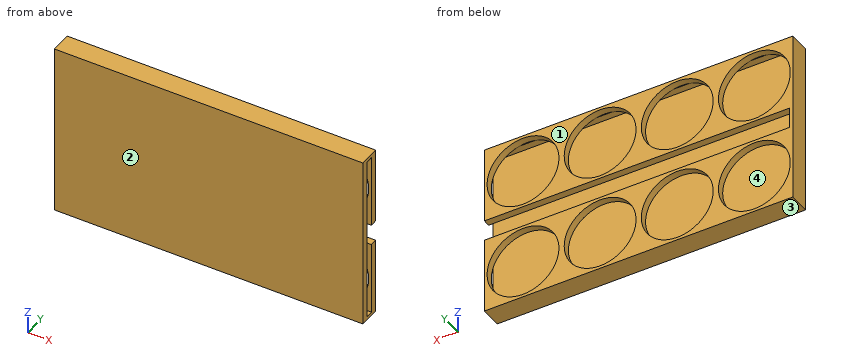
from build123d import *

# Parameters (mm, degrees)
SKETCH1_W           = 88
SKETCH1_H           = 50
BOSS_EXTRUDE1_DEPTH = 6
SKETCH2_W           = 48
SKETCH2_H           = 2
CUT_EXTRUDE1_DEPTH  = 87
SKETCH3_R           = 10.25
CUT_EXTRUDE2_DEPTH  = 2
LPATTERN1_COUNT     = 4
LPATTERN1_PITCH     = 22
SKETCH4_R           = 10.25
CUT_EXTRUDE3_DEPTH  = 2
LPATTERN2_COUNT     = 4
LPATTERN2_PITCH     = 22
SKETCH5_W           = 87
SKETCH5_H           = 6
CUT_EXTRUDE4_DEPTH  = 2


with BuildPart() as part:
    # Sketch1 → Boss-Extrude1 (new body)
    with BuildSketch(Plane(origin=(0, 0, 0), x_dir=(1, 0, 0), z_dir=(0, 1, 0))):
        with Locations((44, 25)):
            Rectangle(SKETCH1_W, SKETCH1_H)
    extrude(amount=-BOSS_EXTRUDE1_DEPTH)

    # Sketch2 → Cut-Extrude1 (cut)
    with BuildSketch(Plane(origin=(88, 0, 0), x_dir=(0, 0, -1), z_dir=(1, 0, 0))):
        with Locations((25, -3)):
            Rectangle(SKETCH2_W, SKETCH2_H)
    extrude(amount=-CUT_EXTRUDE1_DEPTH, mode=Mode.SUBTRACT)

    # Sketch3 → Cut-Extrude2 (cut)
    with BuildSketch(Plane(origin=(0, 0, 0), x_dir=(1, 0, 0), z_dir=(0, 1, 0))):
        with Locations((77, 11)):
            Circle(SKETCH3_R)
    cut_extrude2 = extrude(amount=-CUT_EXTRUDE2_DEPTH, mode=Mode.SUBTRACT)

    # LPattern1: Cut-Extrude2 ×4
    with Locations(*[(-i * LPATTERN1_PITCH, 0, 0) for i in range(1, LPATTERN1_COUNT)]):
        add(cut_extrude2, mode=Mode.SUBTRACT)

    # Sketch4 → Cut-Extrude3 (cut)
    with BuildSketch(Plane(origin=(0, 0, 0), x_dir=(1, 0, 0), z_dir=(0, 1, 0))):
        with Locations((77, 39)):
            Circle(SKETCH4_R)
    cut_extrude3 = extrude(amount=-CUT_EXTRUDE3_DEPTH, mode=Mode.SUBTRACT)

    # LPattern2: Cut-Extrude3 ×4
    with Locations(*[(-i * LPATTERN2_PITCH, 0, 0) for i in range(1, LPATTERN2_COUNT)]):
        add(cut_extrude3, mode=Mode.SUBTRACT)

    # Sketch5 → Cut-Extrude4 (cut)
    with BuildSketch(Plane(origin=(0, 0, 0), x_dir=(1, 0, 0), z_dir=(0, 1, 0))):
        with Locations((44.5, 25)):
            Rectangle(SKETCH5_W, SKETCH5_H)
    extrude(amount=-CUT_EXTRUDE4_DEPTH, mode=Mode.SUBTRACT)


solid = part.part
The model under review builds one solid part; all positions refer to its coordinate system, in mm. Face numbers are marked on the shaded views. Coordinates: 2 decimals unless noted, no trailing zeros. Write each loop counter-clockwise with the first axis right and the second up, starting at its lowest first coordinate (ties: lowest second). Pieces come first, ordered by that corner, then holes. Notation, with made-up numbers: (51, 42.5) - (81, 42.5) arc R14 cw to (81, 52.5) - close; hole circle Ø2 at (84.25, 74). An arc over 180 degrees is marked (long way). Answer as a JSON object with one key per item and string values. Group by question number.
1. Mouldability with a two-part tool opening along Y and no side actions: class the marked faces 1, 2, 3 and 4 as pulls with the +Y half, pulls with the -Y half, needs draft (parallel to the pull), parting line crosses it, or undercut.
2. Add section D-D (z = -32). Give the boundary of the cut face in (x, y), plus the area to 3 significant figures.
3. Add section B-B (z = -11). Give the boundary of the cut face in (x, y).
4. Clearance check with a flat-ended pin moving along its axis: pin 1 Ø2 at (x, z) = (22, -25) entering from +Y. State where the tip first meets the part, or that it passes through.
5. Add section A-A (x = 11). Give the boundary of the cut face in (y, z).
6. To check wall thickness, follow probe 1 along Z at (x, y) = (77, -1.35); probe 2 along X at (y, z) = (-1.5, -10.5); probe 3 along Y at (x, z) = (23, -18). State the ranges of each line that lie inside material, in increasing order.
7. Add section C-C (y = -1). Give the number of separate pieces and of enclosed holes in the cut face, plus the area to 3 significant figures.
Findings:
{
 "1": {"face 1": "pulls with the +Y half", "face 2": "pulls with the -Y half", "face 3": "needs draft", "face 4": "undercut"},
 "2": {"outline": "(0, -6) - (88, -6) - (88, -4) - (1, -4) - (1, -2) - (3.51, -2) - (3.51, 0) - (0, 0) - close; (18.49, -2) - (25.51, -2) - (25.51, 0) - (18.49, 0) - close; (40.49, -2) - (47.51, -2) - (47.51, 0) - (40.49, 0) - close; (62.49, -2) - (69.51, -2) - (69.51, 0) - (62.49, 0) - close; (84.49, -2) - (88, -2) - (88, 0) - (84.49, 0) - close", "area": "234 mm²"},
 "3": {"outline": "(0, -6) - (88, -6) - (88, -4) - (1, -4) - (1, -2) - (0.75, -2) - (0.75, 0) - (0, 0) - close; (21.25, -2) - (22.75, -2) - (22.75, 0) - (21.25, 0) - close; (43.25, -2) - (44.75, -2) - (44.75, 0) - (43.25, 0) - close; (65.25, -2) - (66.75, -2) - (66.75, 0) - (65.25, 0) - close; (87.25, -2) - (88, -2) - (88, 0) - (87.25, 0) - close"},
 "4": {"pin 1": "y = -4"},
 "5": {"outline": "(-6, -50) - (0, -50) - (0, -49.25) - (-2, -49.25) - (-2, -49) - (-4, -49) - (-4, -1) - (-2, -1) - (-2, -0.75) - (0, -0.75) - (0, 0) - (-6, 0) - close; (-2, -28.75) - (0, -28.75) - (0, -28) - (-2, -28) - close; (-2, -22) - (0, -22) - (0, -21.25) - (-2, -21.25) - close"},
 "6": {"probe 1": "-50 to -49.25, -28.75 to -28, -22 to -21.25, -0.75 to 0", "probe 2": "0 to 0.76, 21.24 to 22.76, 43.24 to 44.76, 65.24 to 66.76, 87.24 to 88", "probe 3": "-6 to -4, -2 to 0"},
 "7": {"separate pieces": "1", "enclosed holes": "8", "area": "1,240 mm²"}
}
